Verification items for this drawing (mm, ordinates from the low corner). Give positions to 0.01 mm unless a question says otherwise; leave off trailing zeros. Write each loop counter-clockwise with the first axis right and the second up, starting at its lowest first coordinate (ties: lowest second). Pieces come first, ordered by that corner, then holes. Notation, with made-up numbers: (-25.75, 36) -> (16.25, 36) arc R5 ccw to (16.25, 44) -> close; hole circle Ø1 at (79.5, 66.5). An arc over 180 degrees is marked (long way). One line per item, written item: value.
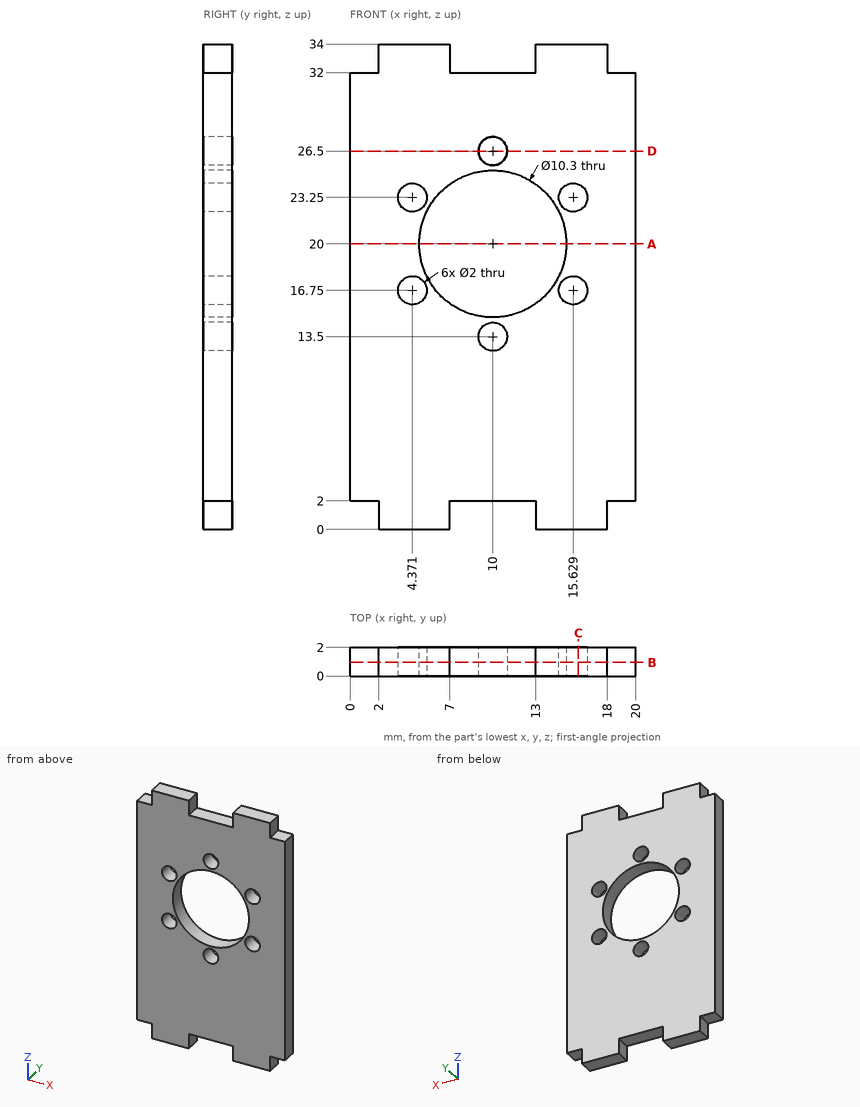
1) Sectioned sample at C-C on x = 16. Record the cut outline in (y, z).
Verdict:
outline: (0, 0) -> (2, 0) -> (2, 15.82) -> (0, 15.82) -> close; (0, 17.68) -> (2, 17.68) -> (2, 22.32) -> (0, 22.32) -> close; (0, 24.18) -> (2, 24.18) -> (2, 34) -> (0, 34) -> close
2) Depth check by flat-ended pin: pin 1 Ø0.6 at (x, y) = (0.5, 0.5) entering from +Z; pin 2 Ø1 at (y, z) = (1.5, 33) entering from -X. Enter the tip coordinate at first touch or a pass-through.
Verdict:
pin 1: z = 32
pin 2: x = 2
3) Sectioned sample at B-B on y = 0.95. Record the cut outline in (x, z), plus the area to 3 significant figures.
Verdict:
outline: (0, 2) -> (2, 2) -> (2, 0) -> (7, 0) -> (7, 2) -> (13, 2) -> (13, 0) -> (18, 0) -> (18, 2) -> (20, 2) -> (20, 32) -> (18, 32) -> (18, 34) -> (13, 34) -> (13, 32) -> (7, 32) -> (7, 34) -> (2, 34) -> (2, 32) -> (0, 32) -> close; hole circle Ø2 at (4.37, 16.75); hole circle Ø2 at (4.37, 23.25); hole circle Ø10.3 at (10, 20); hole circle Ø2 at (10, 13.5); hole circle Ø2 at (10, 26.5); hole circle Ø2 at (15.63, 16.75); hole circle Ø2 at (15.63, 23.25)
area: 538 mm^2
4) Sectioned sample at A-A on z = 20. Record the cut outline in (x, y), plus the area to 3 significant figures.
Verdict:
outline: (0, 0) -> (4.85, 0) -> (4.85, 2) -> (0, 2) -> close; (15.15, 0) -> (20, 0) -> (20, 2) -> (15.15, 2) -> close
area: 19.4 mm^2
5) Scan lines: probe 1 along Z at (x, y) = (10, 1.1); probe 2 along Z at (x, y) = (4.5, 1.35); probe 3 along Z at (x, y) = (16.5, 1.3). Record each from-to range of solid material in increasing order.
Verdict:
probe 1: 2 to 12.5, 14.5 to 14.85, 25.15 to 25.5, 27.5 to 32
probe 2: 0 to 15.76, 17.74 to 22.26, 24.24 to 34
probe 3: 0 to 16.26, 17.24 to 22.76, 23.74 to 34
6) Sectioned sample at D-D on z = 26.5. Record the cut outline in (x, y).
Verdict:
outline: (0, 0) -> (9, 0) -> (9, 2) -> (0, 2) -> close; (11, 0) -> (20, 0) -> (20, 2) -> (11, 2) -> close
